```python
from build123d import *

# Parameters (mm, degrees)
SALIENTE_EXTRUIR1_DEPTH = 3.2
CORTAR_EXTRUIR1_DEPTH   = 3.2
REDONDEO1_R             = 3
CROQUIS3_R              = 2.05
CORTAR_EXTRUIR2_DEPTH   = 3.2
CORTAR_EXTRUIR3_DEPTH   = 3.2
CROQUIS5_R              = 1.55
CORTAR_EXTRUIR4_DEPTH   = 3.2
CROQUIS6_W              = 3
CROQUIS6_H              = 0.2
CORTAR_EXTRUIR5_DEPTH   = 3.2


with BuildPart() as part:
    # Croquis1 → Saliente-Extruir1 (new body)
    with BuildSketch(Plane(origin=(0, 0, 0), x_dir=(1, 0, 0), z_dir=(0, 1, 0))):
        Polygon((7, 65.9), (10, 65.9), (10, 62.7), (7, 62.7), (7, 61.3), (3, 61.3), (3, 62.7), (0, 62.7), (0, 56.8), (-3, 56.8), (-3, 51), (0, 51), (0, 0), (165, 0), (165, 1.5), (168, 1.5), (168, 7.5), (165, 7.5), (165, 13.4), (162, 13.4), (162, 12), (158, 12), (158, 13.4), (155, 13.4), (155, 16.6), (158, 16.6), (158, 18), (162, 18), (162, 16.6), (165, 16.6), (165, 22.5), (168, 22.5), (168, 28.5), (165, 28.5), (165, 377), (30, 377), (30, 373.9), (21.6, 373.9), (21.6, 370.9), (23, 370.9), (23, 366.9), (21.6, 366.9), (21.6, 363.9), (18.4, 363.9), (18.4, 366.9), (17, 366.9), (17, 370.9), (18.4, 370.9), (18.4, 373.9), (10, 373.9), (10, 377), (0, 377), (0, 357.6), (-3, 357.6), (-3, 351.8), (0, 351.8), (0, 345.9), (3, 345.9), (3, 347.3), (7, 347.3), (7, 345.9), (10, 345.9), (10, 342.7), (7, 342.7), (7, 341.3), (3, 341.3), (3, 342.7), (0, 342.7), (0, 336.8), (-3, 336.8), (-3, 331), (0, 331), (0, 217.6), (-3, 217.6), (-3, 211.8), (0, 211.8), (0, 205.9), (3, 205.9), (3, 207.3), (7, 207.3), (7, 205.9), (10, 205.9), (10, 202.7), (7, 202.7), (7, 201.3), (3, 201.3), (3, 202.7), (0, 202.7), (0, 196.8), (-3, 196.8), (-3, 191), (0, 191), (0, 77.6), (-3, 77.6), (-3, 71.8), (0, 71.8), (0, 65.9), (3, 65.9), (3, 67.3), (7, 67.3), align=None)
    extrude(amount=SALIENTE_EXTRUIR1_DEPTH)

    # Croquis2 → Cortar-Extruir1 (cut)
    with BuildSketch(Plane.XZ):
        with BuildLine():
            Line((165, -377), (33, -377))
            ThreePointArc((33, -377), (68.343071274, -192.304293087), (165, -31))
            Line((165, -31), (165, -377))
        make_face()
    extrude(amount=-CORTAR_EXTRUIR1_DEPTH, mode=Mode.SUBTRACT)

    # Redondeo1
    redondeo1_edges = [part.edges().sort_by_distance(p)[0] for p in [
        (33, 1.6, -377),
    ]]
    fillet(redondeo1_edges, radius=REDONDEO1_R)

    # Croquis3 → Cortar-Extruir2 (cut)
    with BuildSketch(Plane(origin=(0, 3.2, 0), x_dir=(1, 0, 0), z_dir=(0, 1, 0))):
        with Locations(Location((40, 80, 0), (0, 0, 270))):
            Circle(CROQUIS3_R)
        with Locations(Location((90, 80, 0), (0, 0, 270))):
            Circle(CROQUIS3_R)
        with Locations(Location((40, 230, 0), (0, 0, 270))):
            Circle(CROQUIS3_R)
    extrude(amount=-CORTAR_EXTRUIR2_DEPTH, mode=Mode.SUBTRACT)

    # Croquis4 → Cortar-Extruir3 (cut)
    with BuildSketch(Plane.XZ):
        with BuildLine():
            Line((143, -30.5), (129, -30.5))
            ThreePointArc((129, -30.5), (127.585786438, -31.085786438), (127, -32.5))
            Line((127, -32.5), (127, -38.5))
            ThreePointArc((127, -38.5), (127.585786438, -39.914213562), (129, -40.5))
            Line((129, -40.5), (143, -40.5))
            ThreePointArc((143, -40.5), (144.414213562, -39.914213562), (145, -38.5))
            Line((145, -38.5), (145, -32.5))
            ThreePointArc((145, -32.5), (144.414213562, -31.085786438), (143, -30.5))
        make_face()
    extrude(amount=-CORTAR_EXTRUIR3_DEPTH, mode=Mode.SUBTRACT)

    # Croquis5 → Cortar-Extruir4 (cut)
    with BuildSketch(Plane.XZ):
        with Locations(Location((110, -95, 0), (0, 0, 270))):
            Circle(CROQUIS5_R)
        with Locations(Location((35, -95, 0), (0, 0, 270))):
            Circle(CROQUIS5_R)
        with Locations(Location((15, -175, 0), (0, 0, 270))):
            Circle(CROQUIS5_R)
        with Locations(Location((60, -175, 0), (0, 0, 270))):
            Circle(CROQUIS5_R)
        with Locations(Location((77, -35.5, 0), (0, 0, 270))):
            Circle(CROQUIS5_R)
        with Locations(Location((37, -215.5, 0), (0, 0, 270))):
            Circle(CROQUIS5_R)
        with Locations(Location((57, -155.5, 0), (0, 0, 270))):
            Circle(CROQUIS5_R)
    extrude(amount=-CORTAR_EXTRUIR4_DEPTH, mode=Mode.SUBTRACT)

    # Croquis6 → Cortar-Extruir5 (cut)
    with BuildSketch(Plane.XZ):
        with Locations((-1.5, -357.5)):
            Rectangle(CROQUIS6_W, CROQUIS6_H)
        with Locations((-1.5, -351.9)):
            Rectangle(CROQUIS6_W, CROQUIS6_H)
        with Locations((-1.5, -336.7)):
            Rectangle(CROQUIS6_W, CROQUIS6_H)
        with Locations((-1.5, -331.1)):
            Rectangle(CROQUIS6_W, CROQUIS6_H)
        with Locations((-1.5, -217.5)):
            Rectangle(CROQUIS6_W, CROQUIS6_H)
        with Locations((-1.5, -211.9)):
            Rectangle(CROQUIS6_W, CROQUIS6_H)
        with Locations((-1.5, -196.7)):
            Rectangle(CROQUIS6_W, CROQUIS6_H)
        with Locations((-1.5, -191.1)):
            Rectangle(CROQUIS6_W, CROQUIS6_H)
        with Locations((-1.5, -77.5)):
            Rectangle(CROQUIS6_W, CROQUIS6_H)
        with Locations((-1.5, -71.9)):
            Rectangle(CROQUIS6_W, CROQUIS6_H)
        with Locations((-1.5, -56.7)):
            Rectangle(CROQUIS6_W, CROQUIS6_H)
        with Locations((-1.5, -51.1)):
            Rectangle(CROQUIS6_W, CROQUIS6_H)
        with Locations((166.5, -28.4)):
            Rectangle(CROQUIS6_W, CROQUIS6_H)
        with Locations((166.5, -22.6)):
            Rectangle(CROQUIS6_W, CROQUIS6_H)
        with Locations((166.5, -7.4)):
            Rectangle(CROQUIS6_W, CROQUIS6_H)
        with Locations((166.5, -1.6)):
            Rectangle(CROQUIS6_W, CROQUIS6_H)
    extrude(amount=-CORTAR_EXTRUIR5_DEPTH, mode=Mode.SUBTRACT)


solid = part.part
```
Work out the finished part from the listing and answer in its coordinate system (mm). Round coordinates to 2 decimals unless told otherwise and drop trailing zeros. Write each loop counter-clockwise with the first axis right and the second up, starting at its lowest first coordinate (ties: lowest second). Pieces come first, ordered by that corner, then holes. Notation, with made-up numbers: (41.25, 63.5) -> (76.25, 63.5) arc R9 cw to (76.25, 67.5) -> close; hole circle Ø1 at (-17.5, 19). An arc over 180 degrees is marked (long way). Write each question's results on one line, items separated by ' | '.
1) The part is cut by section A-A (y = 0.9). State how many separate pieces and enclosed holes the cut face has, and give its area (3 significant figures).
Findings:
separate pieces: 1 | enclosed holes: 11 | area: 30,800 mm²
2) Flat-ended cylindrical pins translate along their axes: pin 1 (1.6 mm diameter, centred on y = 1, z = -14.5, fed in from +X); pin 2 (1.5 mm diameter, centred on y = 1.5, z = -305.5, fed in from -X); pin 3 (2.5 mm diameter, centred on x = 77, z = -35.5, fed in from -Y). Find the tip coordinate at first contact, or state that the pin passes through.
Findings:
pin 1: stops at x = 155 | pin 2: stops at x = 0 | pin 3: passes through
3) The part is cut by section B-B (x = 99). Write down the section's boundary in (y, z), and give its area (3 significant figures).
Findings:
outline: (0, -125.88) -> (3.2, -125.88) -> (3.2, 0) -> (0, 0) -> close | area: 403 mm²
4) Consider line 1 along X through (y, z) = (2, -35.5); line 2 along X through (y, z) = (1.5, -95); line 3 along X through (y, z) = (2.55, -155.5). Determine where each line is inside the solid, lowest interval first. Write a range as [from, to].
Findings:
line 1: x = [0, 75.45], [78.55, 127], [145, 161.13] | line 2: x = [0, 33.45], [36.55, 108.45], [111.55, 117.24] | line 3: x = [0, 55.45], [58.55, 83.97]
